Model file for the job. Use its own axes, mm. A direction names the side the tool comes from. Round coordinates to 2 decimals unless told otherwise and drop trailing zeros. Order: outer loops, then holes, each group sorted by start corner. A loop starts at its lowest first (then second) coordinate and runs counter-clockwise, first axis right, second up. Notation, with made-up numbers: (32.5, 58.25) - (75.5, 58.25) arc R28 cw to (75.5, 79.25) - close; hole circle Ø2 at (15, -1). An arc over 180 degrees is marked (long way). Use one line per item in the form item = value.
from build123d import *

# Parameters (mm, degrees)
SKETCH1_R                  = 38
BOSS_EXTRUDE1_DEPTH        = 68.5
SKETCH3_R                  = 20.5
CUT_EXTRUDE1_DEPTH         = 2
SKETCH4_R                  = 11
BOSS_EXTRUDE3_DEPTH        = 6.35
CHAMFER1_SIZE              = 4.35
CHAMFER1_SIZE2             = 3.916757593
F_10_32_TAPPED_HOLE1_D     = 4.0386
F_10_32_TAPPED_HOLE1_DEPTH = 5.6
F_10_32_TAPPED_HOLE1_TIP   = 1.213317848
F_10_32_TAPPED_HOLE2_D     = 4.0386
F_10_32_TAPPED_HOLE2_DEPTH = 13
F_10_32_TAPPED_HOLE2_TIP   = 1.213317848


with BuildPart() as part:
    # Sketch1 → Boss-Extrude1 (new body)
    with BuildSketch(Plane.XY):
        Circle(SKETCH1_R)
    extrude(amount=BOSS_EXTRUDE1_DEPTH)

    # Sketch3 → Cut-Extrude1 (cut)
    with BuildSketch(Plane(origin=(0, 0, 0), x_dir=(-1, 0, 0), z_dir=(0, 0, -1))):
        Circle(SKETCH3_R)
    extrude(amount=-CUT_EXTRUDE1_DEPTH, mode=Mode.SUBTRACT)

    # Sketch4 → Boss-Extrude3 (add)
    with BuildSketch(Plane.XY.offset(2)):
        Circle(SKETCH4_R)
    extrude(amount=-BOSS_EXTRUDE3_DEPTH)

    # Chamfer1
    chamfer1_edges = [part.edges().sort_by_distance(p)[0] for p in [
        (-11, 0, -4.35),
    ]]
    chamfer1_side = [part.faces().sort_by_distance(p)[0] for p in [
        (-11, 0, -1.175),
    ]]
    chamfer(chamfer1_edges, length=CHAMFER1_SIZE, length2=CHAMFER1_SIZE2, reference=chamfer1_side[0])

    # #10-32 Tapped Hole1
    with Locations(Plane.XY.offset(68.5)):
        with Locations((0, 0)):
            Hole(F_10_32_TAPPED_HOLE1_D / 2, depth=F_10_32_TAPPED_HOLE1_DEPTH)
            with Locations((0, 0, -(F_10_32_TAPPED_HOLE1_DEPTH + F_10_32_TAPPED_HOLE1_TIP / 2))):  # 118° drill point
                Cone(0, F_10_32_TAPPED_HOLE1_D / 2, F_10_32_TAPPED_HOLE1_TIP, mode=Mode.SUBTRACT)

    # #10-32 Tapped Hole2
    with Locations(Plane(origin=(0, 0, -4.35), x_dir=(-1, 0, 0), z_dir=(0, 0, -1))):
        with Locations((0, 0)):
            Hole(F_10_32_TAPPED_HOLE2_D / 2, depth=F_10_32_TAPPED_HOLE2_DEPTH)
            with Locations((0, 0, -(F_10_32_TAPPED_HOLE2_DEPTH + F_10_32_TAPPED_HOLE2_TIP / 2))):  # 118° drill point
                Cone(0, F_10_32_TAPPED_HOLE2_D / 2, F_10_32_TAPPED_HOLE2_TIP, mode=Mode.SUBTRACT)


solid = part.part
(1) Tool access for faces 4 (the face through (16, -16, 0)), 5 (the face through (-1.926, 0.607, 65.661)), 6 (the face through (-2, -1, -4.35)): list every direction of +Z, -Z, +X, -X, +Y, -Y with a clear straight run to the whole face (end or side of a thin tool).
Report:
face_4 = -Z
face_5 = +Z
face_6 = -Z, +X, -X, +Y, -Y
(2) Slice it at D-D on z = 6.5. Give the cut face in (x, y), then the cut area to 3 significant figures.
Report:
outline = circle Ø76 at (0, 0); hole circle Ø4.04 at (0, 0)
area = 4,520 mm2
(3) Pull direction Y, two halves, no side cores. Call faces 1 (the face through (0.076, -0.342, 9.653)), 2 (the face through (-1, -8, 68.5)), 3 (the face through (17.535, -33.713, 33.77)): released by +Y, released by -Y, zero draft, split by the parting line, or undercut.
Report:
face_1 = undercut
face_2 = zero draft
face_3 = split by the parting line
(4) Slice it at A-A on x = 17.5. Give the cut face in (y, z), then the cut area to 3 significant figures.
Report:
outline = (-33.73, 0) - (-10.68, 0) - (-10.68, 2) - (10.68, 2) - (10.68, 0) - (33.73, 0) - (33.73, 68.5) - (-33.73, 68.5) - close
area = 4,580 mm2
(5) Slice it at C-C on y = -14. Give the cut face in (x, z), then the cut area to 3 significant figures.
Report:
outline = (-35.33, 0) - (-14.97, 0) - (-14.97, 2) - (14.97, 2) - (14.97, 0) - (35.33, 0) - (35.33, 68.5) - (-35.33, 68.5) - close
area = 4,780 mm2
(6) Slice it at B-B on z = 24. Give the cut face in (x, y), then the cut area to 3 significant figures.
Report:
outline = circle Ø76 at (0, 0)
area = 4,540 mm2
(7) Pin check, flat tips, straight feed: pin 1 (1 mm diameter, centred on y = 21.5, z = 11.5, fed in from +X); pin 2 (5 mm diameter, centred on x = -21, y = 0, fed in from -Z); pin 3 (6 mm diameter, centred on x = 10.5, z = 12.5, fed in from -Y). Stop position of each tip, or through.
Report:
pin_1 = 31.67
pin_2 = 0
pin_3 = -37.25
(8) Probe probe 1 along Y at (x, z) = (0, 64.7); probe 2 along X at (y, z) = (7.5, 0.5); probe 3 along Z at (x, y) = (30.5, 0). List the from-to ranges inside material, lowest first. Write a range as [from, to].
Report:
probe_1 = [-38, -2.02], [2.02, 38]
probe_2 = [-37.25, -19.08], [-8.05, 8.05], [19.08, 37.25]
probe_3 = [0, 68.5]
